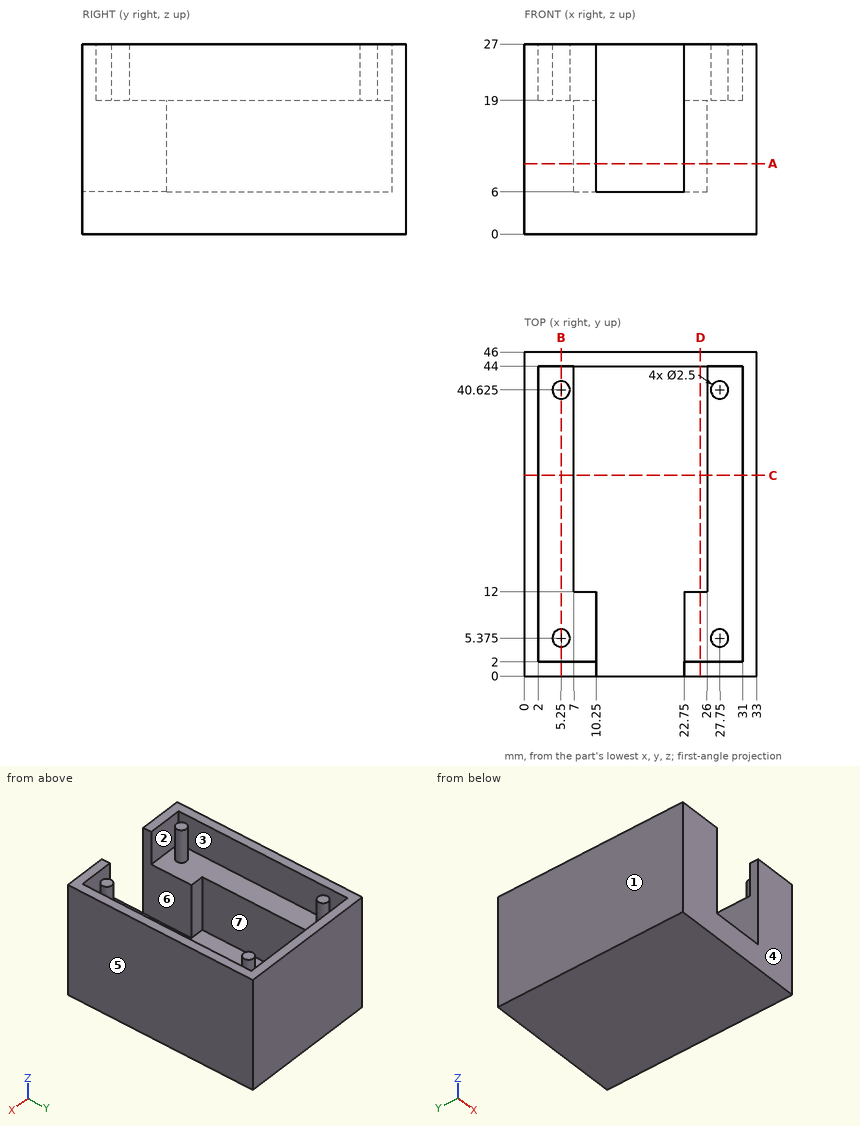
The figure shows three views and two pictorial views of one solid part (mm, origin at its lowest corner). Answer the questions. A direction names the side the tool comes from. Give positions to 0.01 mm unless a question says otherwise; leave off trailing zeros. Loops run counter-clockwise (first coordinate to the right, second up) from the corner with the lowest first, then second, coordinate; pieces in that order, holes last. Notation, with made-up numbers: (-8, 3) -> (10, 3) arc R26 ccw to (10, 19) -> close; hole circle Ø5 at (9.5, 22). An arc over 180 degrees is marked (long way). Put each result on its own line as item: value. Start each with the question number.
Item 1: The part is cut by section D-D (x = 25). Give the vertices of the cut face in (y, z), then the cut area to 3 significant figures.
Item 2: Which of the six approach directions +Z, -Z, +X, -X, +Y, -Y give full straight-line access (tool end or side, diameter ignored) to the marked faces 5, 6 and 7?
Item 3: Each of these flat-tipped pins is pushed along its axis until it touches: P1, Ø9.5, axis at y = 7.5, z = 18.5, coming from the -X side; P2, Ø6.5, axis at x = 8, y = 33, coming from the +Z side; P3, Ø9.5, axis at x = 20, y = 23, coming from the +Z side; P4, Ø1, axis at x = 15, z = 13.5, coming from the -Y side. Where does it stop, or does it pass through?
Item 4: The part is cut by section B-B (x = 5.25). Give the vertices of the cut face in (y, z) (3 decimals), then the cut area to 3 significant figures.
Item 5: The part is cut by section C-C (y = 28.5). Give the vertices of the cut face in (x, z), then the cut area to 3 significant figures.
Item 6: The mould has two halves that part along Y. Classify the marked faces 1, 2, 3 and 4: released by +Y, released by -Y, zero draft, split by the parting line, or undercut.
Item 7: Find the intervals of material crossed by L1, parallel to Y at x = 3, z = 26; L2, parallel to X at y = 35, z = 22.75; L3, parallel to X at y = 40.5, z = 18.5, in increasing order. Write a range as [from, to].
Item 8: The part is cut by section A-A (z = 10). Give the vertices of the cut face in (x, y).
Answers below:
1. outline: (0, 0) -> (46, 0) -> (46, 27) -> (44, 27) -> (44, 6) -> (12, 6) -> (12, 19) -> (2, 19) -> (2, 27) -> (0, 27) -> close
1. area: 490 mm2
2. face 5: +Z, -Z, +X, +Y, -Y
2. face 6: +Z, -Y
2. face 7: +Z
3. P1: x = 0
3. P2: z = 19
3. P3: z = 6
3. P4: y = 44
4. outline: (0, 0) -> (46, 0) -> (46, 27) -> (44, 27) -> (44, 19) -> (41.875, 19) -> (41.875, 27) -> (39.375, 27) -> (39.375, 19) -> (6.625, 19) -> (6.625, 27) -> (4.125, 27) -> (4.125, 19) -> (2, 19) -> (2, 27) -> (0, 27) -> close
4. area: 946 mm2
5. outline: (0, 0) -> (33, 0) -> (33, 27) -> (31, 27) -> (31, 19) -> (26, 19) -> (26, 6) -> (7, 6) -> (7, 19) -> (2, 19) -> (2, 27) -> (0, 27) -> close
5. area: 412 mm2
6. face 1: zero draft
6. face 2: undercut
6. face 3: undercut
6. face 4: released by -Y
7. L1: [0, 2], [44, 46]
7. L2: [0, 2], [31, 33]
7. L3: [0, 7], [26, 33]
8. outline: (0, 0) -> (10.25, 0) -> (10.25, 12) -> (7, 12) -> (7, 44) -> (26, 44) -> (26, 12) -> (22.75, 12) -> (22.75, 0) -> (33, 0) -> (33, 46) -> (0, 46) -> close
